Could you check a few things on this drawing? It's one solid part, dimensions in mm from its lowest x, y, z. Give positions to 0.01 mm unless a question says otherwise; leave off trailing zeros. Order: outer loops, then holes, each group sorted by start corner. A loop starts at its lowest first (then second) coordinate and runs counter-clockwise, first axis right, second up. Notation, with made-up numbers: M 32,1.25 L 70,1.25 A23 cw 70,36.25 Z; hole C 32.25,61.5 d4. An arc over 180 degrees is marked long. Use one line per item in the form item = value. Start each with the question number.
1. I want a section at B-B, the plane x = 50. List the corners of the cut face in (y, z) for me, and give its area (3 significant figures).
2. Will these pins go through, and if not, where does the flat tip stop? P1, Ø10, axis at x = 22.5, z = 28, coming from the +Y side; P2, Ø0.9, axis at y = 4, z = 42.5, coming from the -X side; P3, Ø1.5, axis at x = 35, y = 3.5, coming from the +Z side.
3. I need wall thicknesses on L1, parallel to Z at x = 26, y = 4.1; L2, parallel to X at y = 3.85, z = 26; L3, parallel to Y at x = 17, z = 20.5. Which ranges of each line are inside material? Lowest first, please.
4. I want a section at C-C, the plane z = 42. List the corners of the cut face in (x, y) for me, and give its area (3 significant figures).
5. We'd pull the mould along X, two halves only. Please class the marked faces 1 and 2: +X half, -X half, draft (parallel to the pull), parting line (faces both ways), or undercut.
6. I want a section at A-A, the plane y = 2.75. List the corners of the cut face in (x, z) for me.
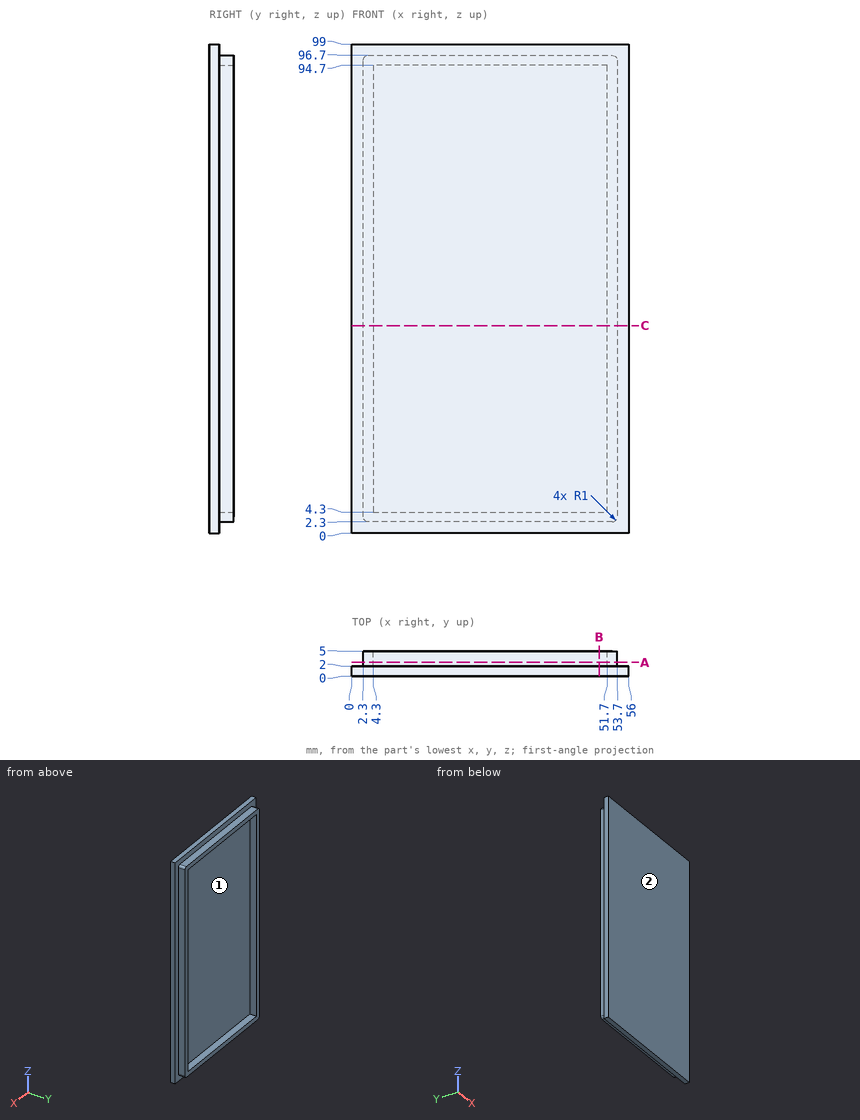
Check result:
q1.outline = M 0,0 L 2,0 L 2,2.3 L 5,2.3 L 5,4.3 L 2,4.3 L 2,94.7 L 5,94.7 L 5,96.7 L 2,96.7 L 2,99 L 0,99 Z
q1.area = 210 mm2
q2.P1 = 2
q2.P2 = 2.3
q2.P3 = 96.7
q3.L1 = 2.3 to 4.3, 94.7 to 96.7
q3.L2 = 2.3 to 4.3, 51.7 to 53.7
q3.L3 = 0 to 2
q4.outline = M 0,0 L 56,0 L 56,2 L 53.7,2 L 53.7,5 L 51.7,5 L 51.7,2 L 4.3,2 L 4.3,5 L 2.3,5 L 2.3,2 L 0,2 Z
q4.area = 124 mm2
q5.face_1 = undercut
q5.face_2 = draft
q6.outline = M 2.3,3.3 A1 ccw 3.3,2.3 L 52.7,2.3 A1 ccw 53.7,3.3 L 53.7,95.7 A1 ccw 52.7,96.7 L 3.3,96.7 A1 ccw 2.3,95.7 Z; hole M 4.3,4.3 L 51.7,4.3 L 51.7,94.7 L 4.3,94.7 Z
